Read the model definition and answer for the solid it produces. Units are mm, in the model's axes. Face numbers are marked on the shaded views. Give positions to 0.01 mm unless a question says otherwise; leave off trailing zeros. Order: outer loops, then holes, each group sorted by start corner. A loop starts at its lowest first (then second) coordinate and runs counter-clockwise, first axis right, second up. Notation, with made-up numbers: (59, 24) -> (110, 24) arc R29 cw to (110, 63) -> close; hole circle Ø11 at (26, 56.5). An arc over 180 degrees is marked (long way). One line per question, with ' | ' between items. Start each with the question number.
```python
from build123d import *

# Parameters (mm, degrees)
SKETCH1_R                                         = 49.5
MAIN_DEPTH                                        = 2
SKETCH2_W                                         = 2.9
SKETCH2_H                                         = 40
SKETCH2_W_2                                       = 2.90180049
MAKERBEAMFIX_DEPTH                                = 1
SKETCH3_W                                         = 9.8
SKETCH3_H                                         = 9.8
CENTRALFIX_DEPTH                                  = 3
CSK_FOR_M2_5_FLAT_HEAD_MACHINE_SCREW1_D           = 3.2
CSK_FOR_M2_5_FLAT_HEAD_MACHINE_SCREW1_CSINK_D     = 6
CSK_FOR_M2_5_FLAT_HEAD_MACHINE_SCREW1_CSINK_ANGLE = 90
SKETCH6_R                                         = 47.5
SKETCH6_R_2                                       = 45.5
CIRCLESUPPORT_DEPTH                               = 2


with BuildPart() as part:
    # Sketch1 → Main (new body)
    with BuildSketch(Plane.XY):
        Circle(SKETCH1_R)
    extrude(amount=MAIN_DEPTH)

    # Sketch2 → MakerBeamFix (add)
    with BuildSketch(Plane.XY.offset(2)):
        with Locations((-10, 0)):
            Rectangle(SKETCH2_W, SKETCH2_H)
        with Locations((10, 0)):
            Rectangle(SKETCH2_W_2, SKETCH2_H)
    extrude(amount=MAKERBEAMFIX_DEPTH)

    # Sketch3 → CentralFix (add)
    with BuildSketch(Plane.XY.offset(2)):
        Rectangle(SKETCH3_W, SKETCH3_H)
    extrude(amount=CENTRALFIX_DEPTH)

    # CSK for M2.5 Flat Head Machine Screw1 (through all)
    with Locations(Plane(origin=(0, 0, 0), x_dir=(-1, 0, 0), z_dir=(0, 0, -1))):
        with Locations((0, 0)):
            CounterSinkHole(CSK_FOR_M2_5_FLAT_HEAD_MACHINE_SCREW1_D / 2, CSK_FOR_M2_5_FLAT_HEAD_MACHINE_SCREW1_CSINK_D / 2, counter_sink_angle=CSK_FOR_M2_5_FLAT_HEAD_MACHINE_SCREW1_CSINK_ANGLE)

    # Sketch6 → CircleSupport (add)
    with BuildSketch(Plane.XY.offset(2)):
        Circle(SKETCH6_R)
        Circle(SKETCH6_R_2, mode=Mode.SUBTRACT)
    extrude(amount=CIRCLESUPPORT_DEPTH)


solid = part.part
```
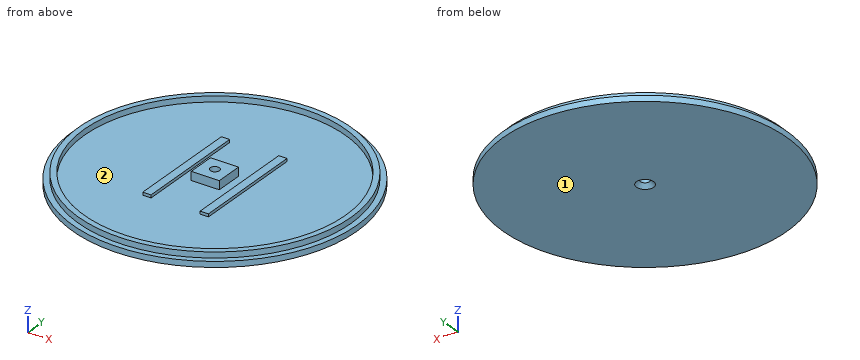
Q1. A cutting plane is placed at D-D, the plane x = -23. Determine the outline of the cut face in (y, z), then the cut area to 3 significant figures.
Q2. Find the intervals of material crossed by line 1 (Y direction, x = 0, z = 2.6); line 2 (X direction, y = -4, z = 2.25); line 3 (Z direction, x = -14, y = -25), in increasing order.
Q3. Given P1, Ø1, axis at x = 6.5, y = 37, coming from the +Z side; P2, Ø0.8, axis at x = 10.5, z = 2.5, coming from the +Y side; P3, Ø0.9, axis at y = 0, z = 4, coming from the +X side; P4, Ø1.9, axis at x = 0, y = 0, coming from the +Z side, each flat-ended and moving along its own axis, determine where each tip first touches the part or whether it passes through.
Q4. Determine the mould class of the marked faces 1 and 2 for opening direction Y: pulls with the +Y half, pulls with the -Y half, needs draft (parallel to the pull), parting line crosses it, or undercut.
Q5. A cutting plane is placed at B-B, the plane x = 0. Determine the outline of the cut face in (y, z).
Q6. A cutting plane is placed at C-C, the plane y = 27. Determine the outline of the cut face in (x, z).
Geometry results:
1) outline: (-43.83, 0) -> (43.83, 0) -> (43.83, 2) -> (41.56, 2) -> (41.56, 4) -> (39.26, 4) -> (39.26, 2) -> (-39.26, 2) -> (-39.26, 4) -> (-41.56, 4) -> (-41.56, 2) -> (-43.83, 2) -> close | area: 185 mm²
2) line 1: -47.5 to -45.5, -4.9 to -1.6, 1.6 to 4.9, 45.5 to 47.5 | line 2: -47.33 to -45.32, -11.45 to -8.55, -4.9 to 4.9, 8.55 to 11.45, 45.32 to 47.33 | line 3: 0 to 2
3) P1: z = 2 | P2: y = 46.41 | P3: x = 47.5 | P4: through
4) face 1: needs draft | face 2: undercut
5) outline: (-49.5, 0) -> (-3, 0) -> (-1.6, 1.4) -> (-1.6, 5) -> (-4.9, 5) -> (-4.9, 2) -> (-45.5, 2) -> (-45.5, 4) -> (-47.5, 4) -> (-47.5, 2) -> (-49.5, 2) -> close; (1.6, 1.4) -> (3, 0) -> (49.5, 0) -> (49.5, 2) -> (47.5, 2) -> (47.5, 4) -> (45.5, 4) -> (45.5, 2) -> (4.9, 2) -> (4.9, 5) -> (1.6, 5) -> close
6) outline: (-41.49, 0) -> (41.49, 0) -> (41.49, 2) -> (39.08, 2) -> (39.08, 4) -> (36.62, 4) -> (36.62, 2) -> (-36.62, 2) -> (-36.62, 4) -> (-39.08, 4) -> (-39.08, 2) -> (-41.49, 2) -> close
